Geometry: final body of the model. Coordinates: model frame, mm. Face numbers are marked on the shaded views. A direction names the side the tool comes from. Round coordinates to 2 decimals unless told otherwise and drop trailing zeros. Loops run counter-clockwise (first coordinate to the right, second up) from the corner with the lowest first, then second, coordinate; pieces in that order, holes last. Notation, with made-up numbers: (38.5, 3.5) - (46.5, 3.5) arc R25 cw to (46.5, 20.5) - close; hole circle Ø9 at (-11.75, -33.5). An arc over 180 degrees is marked (long way). Answer as a JSON object with one key per item and string values. Group by question number.
Item 1: First-contact query: pin 1 (3 mm diameter, centred on x = 13, z = 21, fed in from +Y); pin 2 (18 mm diameter, centred on x = -15.5, z = -4.5, fed in from -Y). Flat tips, straight axial feed; report the tip coordinate or a pass-through.
Item 2: Section B-B (x = 0). Return the cut outline in (y, z), plus the area to 3 significant figures.
Item 3: Line query: line 1 (Z direction, x = -29, y = 203.5); line 2 (X direction, y = 103.5, z = -3); line 3 (Y direction, x = 21.5, z = 14.5). Output: solid intervals per line, ascending.
Item 4: Section A-A (y = 32). Return the cut outline in (x, z).
Item 5: Draft query along Z for the marked faces 1, 2, 3 and 4. Return one class per face: released by +Z, released by -Z, zero draft, split by the parting line, or undercut.
Item 6: Reachability of the marked faces 5, 6 and 7 from +Z, -Z, +X, -X, +Y, -Y: full face, straight path, thin tool, end or side. Return the list, or none.
Item 7: Section C-C (z = 0.5). Return the cut outline in (x, y).
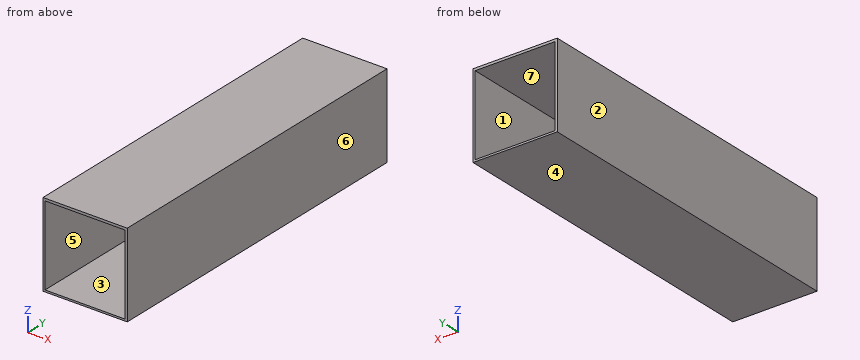
```python
from build123d import *

# Parameters (mm, degrees)
SKETCH1_W           = 63.5
SKETCH1_H           = 63.5
SKETCH1_W_2         = 60.325
SKETCH1_H_2         = 60.325
BOSS_EXTRUDE1_DEPTH = 254
SKETCH3_W           = 60.325
SKETCH3_H           = 60.325
BOSS_EXTRUDE3_DEPTH = 2.54


with BuildPart() as part:
    # Sketch1 → Boss-Extrude1 (new body)
    with BuildSketch(Plane(origin=(0, 0, 0), x_dir=(1, 0, 0), z_dir=(0, 1, 0))):
        with Locations((-4.163673182, -5.031735612)):
            Rectangle(SKETCH1_W, SKETCH1_H)
        with Locations((-4.220828178, -4.80555794)):
            Rectangle(SKETCH1_W_2, SKETCH1_H_2, mode=Mode.SUBTRACT)
    extrude(amount=BOSS_EXTRUDE1_DEPTH)

    # Sketch3 → Boss-Extrude3 (add)
    with BuildSketch(Plane(origin=(0, 152.4, 0), x_dir=(1, 0, 0), z_dir=(0, 1, 0))):
        with Locations((-4.220828178, -4.80555794)):
            Rectangle(SKETCH3_W, SKETCH3_H)
    extrude(amount=-BOSS_EXTRUDE3_DEPTH)


solid = part.part
```
Values:
{
 "1": {"pin 1": "stops at y = 152.4", "pin 2": "stops at y = 149.86"},
 "2": {"outline": "(0, -26.72) - (254, -26.72) - (254, -25.36) - (152.4, -25.36) - (152.4, 34.97) - (254, 34.97) - (254, 36.78) - (0, 36.78) - (0, 34.97) - (149.86, 34.97) - (149.86, -25.36) - (0, -25.36) - close", "area": "960 mm^2"},
 "3": {"line 1": "z = -26.72 to -25.36, 34.97 to 36.78", "line 2": "x = -35.91 to -34.38, 25.94 to 27.59", "line 3": "y = 149.86 to 152.4"},
 "4": {"outline": "(-35.91, -26.72) - (27.59, -26.72) - (27.59, 36.78) - (-35.91, 36.78) - close; hole (-34.38, -25.36) - (25.94, -25.36) - (25.94, 34.97) - (-34.38, 34.97) - close"},
 "5": {"face 1": "undercut", "face 2": "zero draft", "face 3": "undercut", "face 4": "released by -Z"},
 "6": {"face 5": "-Y", "face 6": "+Z, -Z, +X, +Y, -Y", "face 7": "+Y"},
 "7": {"outline": "(-35.91, 0) - (-34.38, 0) - (-34.38, 149.86) - (25.94, 149.86) - (25.94, 0) - (27.59, 0) - (27.59, 254) - (25.94, 254) - (25.94, 152.4) - (-34.38, 152.4) - (-34.38, 254) - (-35.91, 254) - close"}
}
